```python
from build123d import *

# Parameters (mm, degrees)
SM_BASE_FLANGE_1_DEPTH   = 40
CUT_EXTRUDE_1_DEPTH      = 56.072679252
CUT_EXTRUDE_1_DEPTH_BACK = 56.072679252
SKETCH_6_R               = 1.65
CUT_EXTRUDE_3_DEPTH      = 56.072679252
CUT_EXTRUDE_3_DEPTH_BACK = 56.072679252
SKETCH_7_R               = 1.5
SKETCH_7_W               = 56
SKETCH_7_H               = 15
SKETCH_7_W_2             = 38
SKETCH_7_H_2             = 18
CUT_EXTRUDE_2_DEPTH      = 10
FILLET_1_R               = 2


# Sheet-metal steps are written as plain solids
with BuildPart() as part:
    # Sketch 1 → 基体-法兰1 (new, symmetric)
    with BuildSketch(Plane.XY):
        with BuildLine():
            Line((-36, 8), (-36, 1))
            ThreePointArc((-36, 1), (-35.707106781, 0.292893219), (-35, 0))
            Line((-35, 0), (35, 0))
            ThreePointArc((35, 0), (35.707106781, 0.292893219), (36, 1))
            Line((36, 1), (36, 8))
            Line((36, 8), (37, 8))
            Line((37, 8), (37, 1))
            ThreePointArc((37, 1), (36.414213562, -0.414213562), (35, -1))
            Line((35, -1), (-35, -1))
            ThreePointArc((-35, -1), (-36.414213562, -0.414213562), (-37, 1))
            Line((-37, 1), (-37, 8))
            Line((-37, 8), (-36, 8))
        make_face()
    extrude(amount=SM_BASE_FLANGE_1_DEPTH, both=True)

    # 草图6 → 切除-拉伸1 (cut, two sides: drawn at the far end of the back side and taken through both)
    with BuildSketch(Plane(origin=(0, 0, 0), x_dir=(0, 0, -1), z_dir=(1, 0, 0)).offset(-CUT_EXTRUDE_1_DEPTH_BACK)):
        with Locations((-35, 4.5)):
            Circle(SKETCH_6_R)
        with Locations((35, 4.5)):
            Circle(SKETCH_6_R)
        with Locations((0, 4.5)):
            Circle(SKETCH_6_R)
    extrude(amount=CUT_EXTRUDE_1_DEPTH + CUT_EXTRUDE_1_DEPTH_BACK, mode=Mode.SUBTRACT)

    # 草图8 → 切除-拉伸3 (cut, two sides: drawn at the far end of the back side and taken through both)
    with BuildSketch(Plane(origin=(0, 0, 0), x_dir=(0, 0, -1), z_dir=(1, 0, 0)).offset(-CUT_EXTRUDE_3_DEPTH_BACK)):
        with BuildLine():
            Line((-28, 6.5), (-7, 6.5))
            ThreePointArc((-7, 6.5), (-5, 4.5), (-7, 2.5))
            Line((-7, 2.5), (-28, 2.5))
            ThreePointArc((-28, 2.5), (-30, 4.5), (-28, 6.5))
        make_face()
        with BuildLine():
            Line((28, 6.5), (7, 6.5))
            ThreePointArc((7, 6.5), (5, 4.5), (7, 2.5))
            Line((7, 2.5), (28, 2.5))
            ThreePointArc((28, 2.5), (30, 4.5), (28, 6.5))
        make_face()
    extrude(amount=CUT_EXTRUDE_3_DEPTH + CUT_EXTRUDE_3_DEPTH_BACK, mode=Mode.SUBTRACT)

    # 草图7 → 切除-拉伸2 (cut)
    with BuildSketch(Plane.XZ.offset(1)):
        with Locations(Location((19, 17, 0), (0, 0, 270))):
            Circle(SKETCH_7_R)
        with Locations(Location((-19, 17, 0), (0, 0, 270))):
            Circle(SKETCH_7_R)
        with BuildLine():
            Line((-24.75, 31), (-24.75, -16))
            ThreePointArc((-24.75, -16), (-28.75, -20), (-32.75, -16))
            Line((-32.75, -16), (-32.75, 31))
            ThreePointArc((-32.75, 31), (-28.75, 35), (-24.75, 31))
        make_face()
        with BuildLine():
            Line((-13.25, 9), (-13.25, -16))
            ThreePointArc((-13.25, -16), (-17.25, -20), (-21.25, -16))
            Line((-21.25, -16), (-21.25, 9))
            ThreePointArc((-21.25, 9), (-17.25, 13), (-13.25, 9))
        make_face()
        with BuildLine():
            Line((-1.75, 9), (-1.75, -16))
            ThreePointArc((-1.75, -16), (-5.75, -20), (-9.75, -16))
            Line((-9.75, -16), (-9.75, 9))
            ThreePointArc((-9.75, 9), (-5.75, 13), (-1.75, 9))
        make_face()
        with BuildLine():
            Line((21.25, 9), (21.25, -16))
            ThreePointArc((21.25, -16), (17.25, -20), (13.25, -16))
            Line((13.25, -16), (13.25, 9))
            ThreePointArc((13.25, 9), (17.25, 13), (21.25, 9))
        make_face()
        with BuildLine():
            Line((32.75, 31), (32.75, -16))
            ThreePointArc((32.75, -16), (28.75, -20), (24.75, -16))
            Line((24.75, -16), (24.75, 31))
            ThreePointArc((24.75, 31), (28.75, 35), (32.75, 31))
        make_face()
        with Locations((0, -32.5)):
            Rectangle(SKETCH_7_W, SKETCH_7_H)
        with BuildLine():
            Line((9.75, 9), (9.75, -16))
            ThreePointArc((9.75, -16), (5.75, -20), (1.75, -16))
            Line((1.75, -16), (1.75, 9))
            ThreePointArc((1.75, 9), (5.75, 13), (9.75, 9))
        make_face()
        with Locations((0, 31)):
            Rectangle(SKETCH_7_W_2, SKETCH_7_H_2)
    extrude(amount=-CUT_EXTRUDE_2_DEPTH, mode=Mode.SUBTRACT)

    # 圆角1
    fillet_1_edges = [part.edges().sort_by_distance(p)[0] for p in [
        (-36.5, 8, -40),
        (36.5, 8, -40),
        (-28, -0.5, -40),
        (-28, -0.5, -25),
        (28, -0.5, -25),
        (28, -0.5, -40),
        (-19, -0.5, 22),
        (-19, -0.5, 40),
        (19, -0.5, 40),
        (19, -0.5, 22),
        (-36.5, 8, 40),
        (36.5, 8, 40),
    ]]
    fillet(fillet_1_edges, radius=FILLET_1_R)


solid = part.part
```
Work out the finished part from the listing and answer in its coordinate system (mm). A direction names the side the tool comes from. Give positions to 0.01 mm unless a question says otherwise; leave off trailing zeros. Loops run counter-clockwise (first coordinate to the right, second up) from the corner with the lowest first, then second, coordinate; pieces in that order, holes last. Notation, with made-up numbers: (37, 85) -> (51, 85) arc R17 cw to (51, 98) -> close; hole circle Ø9 at (12, -7.5). An arc over 180 degrees is marked (long way). Put each result on its own line as item: value. Start each with the question number.
Item 1: The mould has two halves that part along X. Classify faces 1 (the face through (-5.8, -0.5, 13)), 2 (the face through (-36.5, 4.5, 30)), 3 (the face through (-37, 3, 1)): released by +X, released by -X, zero draft, split by the parting line, or undercut.
Item 2: Find the intervals of material crossed by L1, parallel to X at y = 6.75, z = 22; L2, parallel to Z at x = 36.45, y = 4.5; L3, parallel to Z at x = 18, y = -0.25, in increasing order. Write a range as [from, to].
Item 3: The part is cut by section C-C (x = 31). Give the vertices of the cut face in (y, z), then the cut area to 3 significant figures.
Item 4: Each of these flat-tipped pins is pushed along its axis until it touches: P1, Ø1.1, axis at y = -0.5, z = 28, coming from the +X side; P2, Ø0.5, axis at x = -36.5, z = 18, coming from the -Y side; P3, Ø2, axis at x = 0, z = -25, coming from the +Y side. Where does it stop, or does it pass through?
Item 5: The part is cut by section B-B (z = -31.5). Give the vertices of the cut face in (x, y).
Item 6: Which of the six approach directions +Z, -Z, +X, -X, +Y, -Y give full straight-line access (tool end or side, diameter ignored) to faces 4 (the face through (36.5, 4.5, -30)), 5 (the face through (18.43, -0.49, 22.6)), 6 (the face through (-28.6, -0.49, -39.43)), 7 (the face through (-28.7, -0.5, -20))?
Item 7: The part is cut by section A-A (z = 27). State how many separate pieces and enclosed holes the cut face has, then the cut area to 3 significant figures.
Answers below:
1. face 1: undercut
1. face 2: zero draft
1. face 3: released by -X
2. L1: [-37, -36], [36, 37]
2. L2: [-40, -36.65], [-33.35, -30], [-5, -1.65], [1.65, 5], [30, 33.35], [36.65, 40]
2. L3: [-25, -19.93], [12.93, 15.88], [18.12, 22.27]
3. outline: (-1, -40) -> (0, -40) -> (0, -19.31) -> (-1, -19.31) -> close; (-1, 34.31) -> (0, 34.31) -> (0, 40) -> (-1, 40) -> close
3. area: 26.4 mm2
4. P1: x = 36.76
4. P2: y = -0.56
4. P3: y = 0
5. outline: (-37, 1) arc R2 ccw to (-35, -1) -> (-28, -1) -> (-28, 0) -> (-35, 0) arc R1 cw to (-36, 1) -> (-36, 8) -> (-37, 8) -> close; (28, -1) -> (35, -1) arc R2 ccw to (37, 1) -> (37, 8) -> (36, 8) -> (36, 1) arc R1 cw to (35, 0) -> (28, 0) -> close
6. face 4: +X, -X
6. face 5: +Z, +Y, -Y
6. face 6: -Z, +Y, -Y
6. face 7: +Y, -Y
7. separate pieces: 6
7. enclosed holes: 0
7. area: 26.7 mm2
